Read the model definition and answer for the solid it produces. Units are mm, in the model's axes. Face numbers are marked on the shaded views. A direction names the side the tool comes from. Coordinates: 2 decimals unless noted, no trailing zeros. Write each loop counter-clockwise with the first axis right and the second up, starting at its lowest first coordinate (ties: lowest second). Pieces come first, ordered by that corner, then holes.
(1) Given pin 1 (8 mm diameter, centred on x = 51.14, y = 41.14, fed in from +Z), flat-ended and moving along its own axis, determine where the tip first touches the part or whether it passes through.
(2) Section D-D on y = 4 is taken. Write down the section's boundary in (x, z).
(3) Find the intervals of material crossed by probe 1 along Y at (x, z) = (7, 5); probe 2 along Y at (x, z) = (74, 5.5); probe 3 along Y at (x, z) = (4, 5), in increasing order.
(4) The mould has two halves that part along Y. Classify the marked faces 3, 4 and 5: +Y half, -Y half, draft (parallel to the pull), parting line (faces both ways), or undercut.
(5) Which of the six approach directions +Z, -Z, +X, -X, +Y, -Y give full straight-line access (tool end or side, diameter ignored) to the marked faces 1 and 2?
(6) Section A-A on y = 53 is taken. Write down the section's boundary in (x, z).
(7) Section C-C on z = 5.5 is taken. State how many separate pieces and enclosed holes the cut face has, then the cut area to 3 significant figures.
(8) Section B-B on x = 73 is taken. Write down the section's boundary in (y, z).
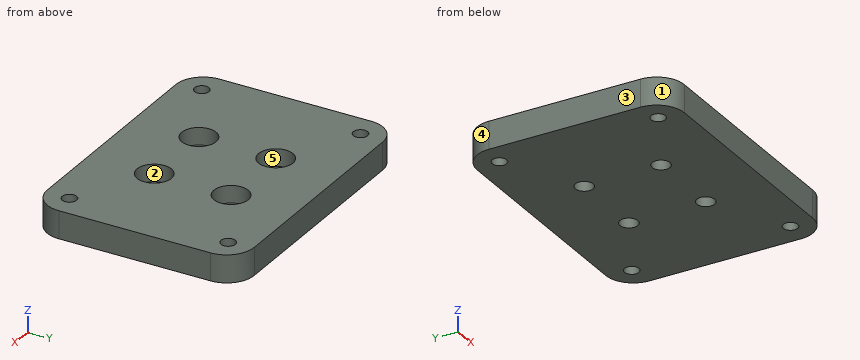
from build123d import *

# Parameters (mm, degrees)
SKETCH_1_W          = 80
SKETCH_1_H          = 60
EXTRUDE_1_DEPTH     = 8
SKETCH_2_R          = 2.6
CUT_EXTRUDE_1_DEPTH = 10
FILLET_1_R          = 8
SKETCH_3_R          = 5
CUT_EXTRUDE_2_DEPTH = 5
SKETCH_5_R          = 2.1
CUT_EXTRUDE_4_DEPTH = 10


with BuildPart() as part:
    # ｽｹｯﾁ1 → ﾎﾞｽ - 押し出し1 (new body)
    with BuildSketch(Plane.XY):
        with Locations((40, 30)):
            Rectangle(SKETCH_1_W, SKETCH_1_H)
    extrude(amount=EXTRUDE_1_DEPTH)

    # ｽｹｯﾁ2 → ｶｯﾄ - 押し出し1 (cut)
    with BuildSketch(Plane.XY.offset(8)):
        with Locations((28.863068196, 41.136931804)):
            Circle(SKETCH_2_R)
        with Locations((51.136931804, 41.136931804)):
            Circle(SKETCH_2_R)
        with Locations((51.136931804, 18.863068196)):
            Circle(SKETCH_2_R)
        with Locations((28.863068196, 18.863068196)):
            Circle(SKETCH_2_R)
    extrude(amount=-CUT_EXTRUDE_1_DEPTH, mode=Mode.SUBTRACT)

    # ﾌｨﾚｯﾄ1
    fillet_1_edges = [part.edges().sort_by_distance(p)[0] for p in [
        (0, 60, 4),
        (80, 60, 4),
        (80, 0, 4),
        (0, 0, 4),
    ]]
    fillet(fillet_1_edges, radius=FILLET_1_R)

    # ｽｹｯﾁ3 → ｶｯﾄ - 押し出し2 (cut)
    with BuildSketch(Plane.XY.offset(8)):
        with Locations((28.863068196, 41.136931804)):
            Circle(SKETCH_3_R)
        with Locations((51.136931804, 41.136931804)):
            Circle(SKETCH_3_R)
        with Locations((28.863068196, 18.863068196)):
            Circle(SKETCH_3_R)
        with Locations((51.136931804, 18.863068196)):
            Circle(SKETCH_3_R)
    extrude(amount=-CUT_EXTRUDE_2_DEPTH, mode=Mode.SUBTRACT)

    # ｽｹｯﾁ5 → ｶｯﾄ - 押し出し4 (cut)
    with BuildSketch(Plane.XY.offset(8)):
        with Locations((7, 53)):
            Circle(SKETCH_5_R)
        with Locations((73, 53)):
            Circle(SKETCH_5_R)
        with Locations((73, 7)):
            Circle(SKETCH_5_R)
        with Locations((7, 7)):
            Circle(SKETCH_5_R)
    extrude(amount=-CUT_EXTRUDE_4_DEPTH, mode=Mode.SUBTRACT)


solid = part.part
Response:
1. pin 1: stops at z = 3
2. outline: (1.07, 0) - (78.93, 0) - (78.93, 8) - (1.07, 8) - close
3. probe 1: y = 0.06 to 4.9, 9.1 to 50.9, 55.1 to 59.94
3. probe 2: y = 0.25 to 5.15, 8.85 to 51.15, 54.85 to 59.75
3. probe 3: y = 1.07 to 58.93
4. face 3: draft
4. face 4: +Y half
4. face 5: undercut
5. face 1: +Z, -Z, -X, -Y
5. face 2: +Z
6. outline: (0.06, 0) - (4.9, 0) - (4.9, 8) - (0.06, 8) - close; (9.1, 0) - (70.9, 0) - (70.9, 8) - (9.1, 8) - close; (75.1, 0) - (79.94, 0) - (79.94, 8) - (75.1, 8) - close
7. separate pieces: 1
7. enclosed holes: 8
7. area: 4,380 mm2
8. outline: (0.06, 0) - (4.9, 0) - (4.9, 8) - (0.06, 8) - close; (9.1, 0) - (50.9, 0) - (50.9, 8) - (9.1, 8) - close; (55.1, 0) - (59.94, 0) - (59.94, 8) - (55.1, 8) - close
